from build123d import *

# Parameters (mm, degrees)
BODY_START           = -10
BODY_DEPTH           = 20
M3_CLEARANCE_HOLE1_D = 3.4
CUT_EXTRUDE1_REACH   = 34.389
SKETCH4_R            = 2.5


# Read off the part's stored shape, not the designer's step: Body
with BuildPart() as part:
    # Body outline → Body (new body)
    with BuildSketch(Plane.XY.offset(BODY_START)):
        Polygon((10, 24.25), (10, 4.25), (-0.5, 4.25), (-0.5, 24.25), (-6.25, 24.25), (-6.25, 4.25), (-12.75, 4.25), (-12.75, -1.25), (12.75, -1.25), (12.75, 24.25), align=None)
    extrude(amount=BODY_DEPTH)

    # M3 Clearance Hole1 (through all)
    with Locations(Plane(origin=(0, -1.25, 0), x_dir=(-1, 0, 0), z_dir=(0, -1, 0))):
        with Locations((9.5, -3), (9.5, 3)):
            Hole(M3_CLEARANCE_HOLE1_D / 2)

    # Cut-Extrude1: up to this face of the body (flat: up to its plane)
    cut_extrude1_end = Plane(part.part.faces().sort_by_distance((12.75, 11.5, 0))[0])
    # Sketch4 → Cut-Extrude1 (cut, up to the picked face)
    with BuildSketch(Plane.ZY.offset(6.25), mode=Mode.PRIVATE) as cut_extrude1_sk1:
        with Locations((0, 14.25)):
            Circle(SKETCH4_R)
    cut_extrude1_tool1 = split(extrude(cut_extrude1_sk1.sketch, amount=-CUT_EXTRUDE1_REACH, mode=Mode.PRIVATE), bisect_by=cut_extrude1_end, keep=Keep.BOTH, mode=Mode.PRIVATE)
    add(cut_extrude1_tool1.solids().sort_by(Axis((-6.25, 14.25, 0), (1, 0, 0)))[0], mode=Mode.SUBTRACT)


solid = part.part
Geometry: final body of the model. Coordinates: model frame, mm. A direction names the side the tool comes from. Coordinates: 2 decimals unless noted, no trailing zeros. Loops run counter-clockwise (first coordinate to the right, second up) from the corner with the lowest first, then second, coordinate; pieces in that order, holes last. Notation, with made-up numbers: (-37, 17) - (-13, 17) arc R10 cw to (-13, 30) - close; hole circle Ø3 at (73.5, 1.25). An arc over 180 degrees is marked (long way). Put each result on its own line as item: value. Start each with the question number.
Q1. Cut plane C-C, the plane x = -9.5. Return loops of the section in (y, z).
Q2. Pull-direction query (Y, two-part tool) for faces 1 (the flat face through (-9, 4.25, 0)), 2 (the cylindrical face through (11.4, 11.8, -0.5)), 3 (the cylindrical face through (-3.4, 11.8, -0.5)), 4 (the flat face through (-0.5, 16, -2)); classes: released by +Y, released by -Y, zero draft, split by the parting line, or undercut.
Q3. Cut plane B-B, the plane z = 3. Return loops of the section in (x, y), and give its area (3 significant figures).
Q4. Cut plane D-D, the plane y = 12.25. Return loops of the section in (x, z), and give its area (4 significant figures).
Q5. Line query: line 1 (Z direction, x = -9.5, y = 1.15); line 2 (Y direction, x = 12, z = 0); line 3 (X direction, y = 15.5, z = 8). Output: solid intervals per line, ascending.
Q6. Pin query (flat end, axial travel): pin 1 Ø2 at (x, y) = (1, 19.5) entering from +Z; pin 2 Ø3 at (y, z) = (12.5, -6) entering from -X; pin 3 Ø8.5 at (x, z) = (5, 0.5) entering from +Y. Return the tip coordinate at first contact, or that it passes through.
Q7. Cut plane A-A, the plane y = 17.75. Return loops of the section in (x, z), and give its area (3 significant figures).
Q8. Set-up query: faces 5 (the flat face through (0, -1.25, 0)), 6 (the flat face through (10, 17, 2)), 7 (the flat face through (-6.25, 17, 2)). Return all of +Z, -Z, +X, -X, +Y, -Y with unobstructed straight access to the full face (end or side cutting, diameter ignored); none if empty.
Filled sheet:
1. outline: (-1.25, -10) - (4.25, -10) - (4.25, -4.7) - (-1.25, -4.7) - close; (-1.25, -1.3) - (4.25, -1.3) - (4.25, 1.3) - (-1.25, 1.3) - close; (-1.25, 4.7) - (4.25, 4.7) - (4.25, 10) - (-1.25, 10) - close
2. face 1: released by +Y
2. face 2: undercut
2. face 3: undercut
2. face 4: zero draft
3. outline: (-12.75, -1.25) - (-11.2, -1.25) - (-11.2, 4.25) - (-12.75, 4.25) - close; (-7.8, -1.25) - (12.75, -1.25) - (12.75, 24.25) - (10, 24.25) - (10, 4.25) - (-0.5, 4.25) - (-0.5, 24.25) - (-6.25, 24.25) - (-6.25, 4.25) - (-7.8, 4.25) - close
3. area: 292 mm²
4. outline: (-6.25, -10) - (-0.5, -10) - (-0.5, -1.5) - (-6.25, -1.5) - close; (-6.25, 1.5) - (-0.5, 1.5) - (-0.5, 10) - (-6.25, 10) - close; (10, -10) - (12.75, -10) - (12.75, -1.5) - (10, -1.5) - close; (10, 1.5) - (12.75, 1.5) - (12.75, 10) - (10, 10) - close
4. area: 144.5 mm²
5. line 1: -10 to -4.7, -1.3 to 1.3, 4.7 to 10
5. line 2: -1.25 to 11.75, 16.75 to 24.25
5. line 3: -6.25 to -0.5, 10 to 12.75
6. pin 1: through
6. pin 2: x = -6.25
6. pin 3: y = 4.25
7. outline: (-6.25, -10) - (-0.5, -10) - (-0.5, 10) - (-6.25, 10) - close; (10, -10) - (12.75, -10) - (12.75, 10) - (10, 10) - close
7. area: 170 mm²
8. face 5: +Z, -Z, +X, -X, -Y
8. face 6: +Z, -Z, +Y
8. face 7: +Z, -Z, -X, +Y
